For this review, take the finished solid that the model builds, in its own axes (mm). A direction names the side the tool comes from. Coordinates: 2 decimals unless noted, no trailing zeros. Write each loop counter-clockwise with the first axis right and the second up, starting at its lowest first coordinate (ties: lowest second). Pieces come first, ordered by that corner, then holes.
1) We need section C-C on x = 82. Write out the cut boundary in (y, z), then the cut area to 3 significant figures.
2) For faces 1 (the face through (-100, 58, -89)), 2 (the face through (45.63, 21.715, -153.735)), 3 (the face through (-1, 85, -180)), list the 3-axis set-ups (+Z, -Z, +X, -X, +Y, -Y) from which the entire face can be reached by the end or side of a thin tool; tool diameter is ignored.
3) To check wall thickness, follow line 1 along X through (y, z) = (45, -154.5); line 2 along X through (y, z) = (75.5, -248.5); line 3 along Y through (x, z) = (59, -281.5). State the ranges of each line that lie inside material, in increasing order.
4) Mouldability with a two-part tool opening along Y and no side actions: class faces 4 (the face through (0.81, 18.47, -314.38)), 5 (the face through (-44.37, 21.4, -153.73)), 6 (the face through (-1, 70, -96)), 7 (the face through (90, 80, -94)) as pulls with the +Y half, pulls with the -Y half, needs draft (parallel to the pull), parting line crosses it, or undercut.
5) We need section D-D on z = -227. Write out the cut boundary in (x, y), then the cut area to 3 significant figures.
6) Insertion check: P1, Ø1.5, axis at x = 43.5, z = -156, coming from the +Y side; P2, Ø16, axis at x = -21, y = 85, coming from the -Z side; P3, Ø10, axis at y = 23.5, z = -283, coming from the -X side. Each pin has a flat end and moves straight along its axis. Give the tip position at first contact, or say it passes through.
7) We need section A-A on z = -28. Write out the cut boundary in (x, y).
8) We need section B-B on y = 38. Write out the cut boundary in (x, z), then the cut area to 3 significant figures.
from build123d import *

# Parameters (mm, degrees)
BOSS_EXTRUDE1_DEPTH = 100
CUT_EXTRUDE1_DEPTH  = 385.317577012
CUT_EXTRUDE2_DEPTH  = 385.317577012
SHELL1_T            = -10
SKETCH5_W           = 180
SKETCH5_H           = 170
BOSS_EXTRUDE4_DEPTH = 40
SKETCH5_3_W         = 180
SKETCH5_3_H         = 170
CUT_EXTRUDE4_DEPTH  = 20
BOSS_EXTRUDE5_DEPTH = 10


with BuildPart() as part:
    # Sketch2 → Boss-Extrude1 (new, symmetric)
    with BuildSketch(Plane(origin=(0, 0, 0), x_dir=(0, 0, -1), z_dir=(1, 0, 0))):
        with BuildLine():
            Line((0, 0), (250, 0))
            ThreePointArc((250, 0), (315.192024052, 18.983962204), (360, 70))
            Line((360, 70), (360, 90))
            Line((360, 90), (0, 90))
            Line((0, 90), (0, 0))
        make_face()
    extrude(amount=BOSS_EXTRUDE1_DEPTH, both=True)

    # Sketch3 → Cut-Extrude1 (cut, through all)
    with BuildSketch(Plane.XY):
        Polygon((0, 0), (-100, 25), (-100, 0), align=None)
        Polygon((100, 0), (100, 25), (0, 0), align=None)
    extrude(amount=-CUT_EXTRUDE1_DEPTH, mode=Mode.SUBTRACT)

    # Sketch4 → Cut-Extrude2 (cut, through all)
    with BuildSketch(Plane(origin=(0, 90, 0), x_dir=(1, 0, 0), z_dir=(0, 1, 0))):
        with BuildLine():
            Line((100, 360), (0, 360))
            ThreePointArc((0, 360), (73.321342538, 282.95630141), (100, 180))
            Line((100, 180), (100, 360))
        make_face()
        with BuildLine():
            Line((-100, 360), (-100, 180))
            ThreePointArc((-100, 180), (-73.321342538, 282.95630141), (0, 360))
            Line((0, 360), (-100, 360))
        make_face()
    extrude(amount=-CUT_EXTRUDE2_DEPTH, mode=Mode.SUBTRACT)

    # Shell1
    shell1_openings = [part.faces().sort_by_distance(p)[0] for p in [
        (0, 90, -156.338581153),
    ]]
    offset(amount=SHELL1_T, openings=shell1_openings)

    # Sketch5 → Boss-Extrude4 (add)
    with BuildSketch(Plane(origin=(0, 90, 0), x_dir=(1, 0, 0), z_dir=(0, 1, 0))):
        with Locations((0, 95)):
            Rectangle(SKETCH5_W, SKETCH5_H)
    extrude(amount=-BOSS_EXTRUDE4_DEPTH)

    # Sketch5<3> → Cut-Extrude4 (cut)
    with BuildSketch(Plane(origin=(0, 90, 0), x_dir=(1, 0, 0), z_dir=(0, 1, 0))):
        with Locations((0, 95)):
            Rectangle(SKETCH5_3_W, SKETCH5_3_H)
    extrude(amount=-CUT_EXTRUDE4_DEPTH, mode=Mode.SUBTRACT)

    # Sketch8 → Boss-Extrude5 (add)
    with BuildSketch(Plane(origin=(0, 90, 0), x_dir=(1, 0, 0), z_dir=(0, 1, 0))):
        with BuildLine():
            Line((-90, 180), (90, 180))
            ThreePointArc((90, 180), (66.084249725, 275.341491492), (0, 348.107108713))
            ThreePointArc((0, 348.107108713), (-66.084249725, 275.341491492), (-90, 180))
        make_face()
    extrude(amount=-BOSS_EXTRUDE5_DEPTH)


solid = part.part
Result:
1. outline: (20.5, -265.49) - (90, -265.49) - (90, -180) - (80, -180) - (80, -236.28) - (30.81, -236.28) - (30.81, -10) - (50, -10) - (50, -180) - (70, -180) - (70, -10) - (90, -10) - (90, 0) - (20.5, 0) - close
1. area: 9,020 mm2
2. face 1: +Z, -Z, -X, +Y, -Y
2. face 2: none
2. face 3: +Y
3. line 1: x = -100 to -90, 90 to 100
3. line 2: x = -88.63 to -78.03, 78.03 to 88.63
3. line 3: y = 14.75 to 25.06, 80 to 90
4. face 4: pulls with the -Y half
4. face 5: undercut
4. face 6: pulls with the +Y half
4. face 7: needs draft
5. outline: (-94.72, 23.68) - (0, 0) - (94.72, 23.68) - (94.72, 90) - (-94.72, 90) - close; hole (-84.46, 31.42) - (0, 10.31) - (84.46, 31.42) - (84.46, 80) - (-84.46, 80) - close
5. area: 4,820 mm2
6. P1: stops at y = 70
6. P2: stops at z = -351.23
6. P3: stops at x = -75.99
7. outline: (-100, 25) - (0, 0) - (100, 25) - (100, 90) - (90, 90) - (90, 70) - (-90, 70) - (-90, 90) - (-100, 90) - close; hole (-90, 32.81) - (0, 10.31) - (90, 32.81) - (90, 50) - (-90, 50) - close
8. outline: (-100, -180) arc R212 ccw to (-29.09, -338.23) - (29.09, -338.23) arc R212 ccw to (100, -180) - (100, 0) - (-100, 0) - close; hole (-90, -180) arc R202 ccw to (-29.8, -323.86) - (29.8, -323.86) arc R202 ccw to (90, -180) - (90, -10) - (-90, -10) - close
8. area: 9,630 mm2
